Part model, mm, in its own coordinate system. A direction names the side the tool comes from. Coordinates: 2 decimals unless noted, no trailing zeros. Loops run counter-clockwise (first coordinate to the right, second up) from the corner with the lowest first, then second, coordinate; pieces in that order, holes last. Notation, with made-up numbers: M 30,82.5 L 42,82.5 A29 cw 42,121.5 Z; hole C -33.75,-30.75 d10. An arc over 180 degrees is marked long. Use a Markdown table: item, result. Add a question column.
1) Tool access for faces 4 (the flat face through (-1, 3, 34.925)), 5 (the conical face through (-26.77, 2.57, 21.29)): list every direction of +Z, -Z, +X, -X, +Y, -Y with a clear straight run to the whole face (end or side of a thin tool).
2) Band-saw the part on D-D (x = 25.4). List the corners of the cut face in (y, z).
3) Band-saw the part on B-B (x = 4). List the corners of the cut face in (y, z) (3 decimals), plus the area to 3 significant figures.
4) Pin check, flat tips, straight feed: pin 1 Ø5 at (x, z) = (11.5, 32) entering from +Y; pin 2 Ø7.5 at (x, z) = (-27.94, 19.05) entering from +Y; pin 3 Ø3 at (y, z) = (2, 6.5) entering from +X. Stop position of each tip, or through.
5) Pull direction Z, two halves, no side cores. Call faces 1 (the flat face through (-9, 0, 2)), 2 (the cylindrical face through (-44.1, 3.13, 38.72)), 3 (the flat face through (17.78, 3, 19)): released by +Z, released by -Z, zero draft, split by the parting line, or undercut.
6) Wall check: probe 1 along X at (y, z) = (3.8, 19.05); probe 2 along X at (y, z) = (4.25, 12); probe 3 along Z at (x, y) = (8, 3.5) (3 decimals). Give the ranges that are in metal, low to high. Write a range as from..to.
7) Band-saw the part on A-A (z = 19.05). List the corners of the cut face in (x, y).
8) Band-saw the part on C-C (z = 31). List the corners of the cut face in (x, y), plus the area to 3 significant figures.
from build123d import *

# Parameters (mm, degrees)
BOSS_EXTRUDE1_DEPTH                             = 6.35
CSK_FOR_10_FLAT_HEAD_MACHINE_SCREW1_D           = 4.826
CSK_FOR_10_FLAT_HEAD_MACHINE_SCREW1_CSINK_D     = 9.525
CSK_FOR_10_FLAT_HEAD_MACHINE_SCREW1_CSINK_ANGLE = 82


with BuildPart() as part:
    # Sketch1 → Boss-Extrude1 (new body)
    with BuildSketch(Plane(origin=(0, 0, 0), x_dir=(1, 0, 0), z_dir=(0, 1, 0))):
        with BuildLine():
            Line((13.97, 6.35), (-30.48, 6.35))
            ThreePointArc((-30.48, 6.35), (-43.950384182, 0.770384182), (-49.53, -12.7))
            Line((-49.53, -12.7), (-49.53, -25.4))
            ThreePointArc((-49.53, -25.4), (-43.950384182, -38.870384182), (-30.48, -44.45))
            Line((-30.48, -44.45), (13.97, -44.45))
            ThreePointArc((13.97, -44.45), (27.440384182, -38.870384182), (33.02, -25.4))
            Line((33.02, -25.4), (33.02, -12.7))
            ThreePointArc((33.02, -12.7), (27.440384182, 0.770384182), (13.97, 6.35))
        make_face()
        with BuildLine():
            Line((-20.32, -12.7), (-20.32, -25.4))
            Line((-20.32, -25.4), (-20.32, -28.575))
            ThreePointArc((-20.32, -28.575), (-18.460128061, -33.065128061), (-13.97, -34.925))
            Line((-13.97, -34.925), (11.43, -34.925))
            ThreePointArc((11.43, -34.925), (15.920128061, -33.065128061), (17.78, -28.575))
            Line((17.78, -28.575), (17.78, -25.4))
            Line((17.78, -25.4), (17.78, -12.7))
            Line((17.78, -12.7), (17.78, -9.525))
            ThreePointArc((17.78, -9.525), (15.920128061, -5.034871939), (11.43, -3.175))
            Line((11.43, -3.175), (-13.97, -3.175))
            ThreePointArc((-13.97, -3.175), (-18.460128061, -5.034871939), (-20.32, -9.525))
            Line((-20.32, -9.525), (-20.32, -12.7))
        make_face(mode=Mode.SUBTRACT)
    extrude(amount=BOSS_EXTRUDE1_DEPTH)

    # CSK for #10 Flat Head Machine Screw1 (through all)
    with Locations(Plane(origin=(0, 0, 0), x_dir=(-1, 0, 0), z_dir=(0, -1, 0))):
        with Locations((27.94, -19.05), (-25.4, -19.05)):
            CounterSinkHole(CSK_FOR_10_FLAT_HEAD_MACHINE_SCREW1_D / 2, CSK_FOR_10_FLAT_HEAD_MACHINE_SCREW1_CSINK_D / 2, counter_sink_angle=CSK_FOR_10_FLAT_HEAD_MACHINE_SCREW1_CSINK_ANGLE)


solid = part.part
Entries:
| question | item | result |
|---|---|---|
| 1 | face 4 | +Y, -Y |
| 1 | face 5 | -Y |
| 2 | outline | M 0,-2.54 L 6.35,-2.54 L 6.35,16.64 L 2.7,16.64 L 0,14.29 Z; M 0,23.81 L 2.7,21.46 L 6.35,21.46 L 6.35,40.64 L 0,40.64 Z |
| 3 | outline | M 0,-6.35 L 6.35,-6.35 L 6.35,3.175 L 0,3.175 Z; M 0,34.925 L 6.35,34.925 L 6.35,44.45 L 0,44.45 Z |
| 3 | area | 121 mm2 |
| 4 | pin 1 | through |
| 4 | pin 2 | y = 6.35 |
| 4 | pin 3 | x = 32.43 |
| 5 | face 1 | zero draft |
| 5 | face 2 | released by +Z |
| 5 | face 3 | undercut |
| 6 | probe 1 | -49.53..-30.35, -25.53..-20.32, 17.78..22.99, 27.81..33.02 |
| 6 | probe 2 | -49.52..-20.32, 17.78..33.01 |
| 6 | probe 3 | -6.35..3.175, 34.925..44.45 |
| 7 | outline | M -49.53,0 L -32.7,0 L -30.35,2.7 L -30.35,6.35 L -49.53,6.35 Z; M -25.53,2.7 L -23.18,0 L -20.32,0 L -20.32,6.35 L -25.53,6.35 Z; M 17.78,0 L 20.64,0 L 22.99,2.7 L 22.99,6.35 L 17.78,6.35 Z; M 27.81,2.7 L 30.16,0 L 33.02,0 L 33.02,6.35 L 27.81,6.35 Z |
| 8 | outline | M -48.69,0 L -19.84,0 L -19.84,6.35 L -48.69,6.35 Z; M 17.3,0 L 32.18,0 L 32.18,6.35 L 17.3,6.35 Z |
| 8 | area | 278 mm2 |
